Study the drawing (mm; zero at the part's minimum x, y, z) and answer. A direction names the side the tool comes from. Round coordinates to 2 decimals unless told otherwise and drop trailing zeros. Write each loop counter-clockwise with the first axis right and the second up, starting at its lowest first coordinate (ties: lowest second). Pieces come first, ordered by that corner, then holes.
(1) A cutting plane is placed at B-B, the plane x = 83. Give the vertices of the cut face in (y, z).
(2) For the marked faces 1, 2 and 3, determine the directions among +Z, -Z, +X, -X, +Y, -Y from which every point of the face is accessible in a straight line to the end or side of a thin tool.
(3) A cutting plane is placed at C-C, the plane z = 7.5. Give the vertices of the cut face in (x, y), and give its area (3 significant figures).
(4) A cutting plane is placed at D-D, the plane x = 113. Give the vertices of the cut face in (y, z), and give its area (3 significant figures).
(5) Find the intervals of material crossed by probe 1 along X at (y, z) = (61, 31.5); probe 2 along X at (y, z) = (65, 18); probe 3 along Z at (x, y) = (142, 99), in increasing order.
(6) The mould has two halves that part along Z. Classify the marked faces 4, 5, 6 and 7: +Z half, -Z half, draft (parallel to the pull), parting line (faces both ways), or undercut.
(7) Each of these flat-tipped pins is pushed along its axis until it touches: pin 1 Ø25 at (x, y) = (16, 94.5) entering from -Z; pin 2 Ø22 at (y, z) = (63, 36) entering from -X; pin 3 Ø6 at (y, z) = (88, 60.5) entering from +X. Where does it stop, or does it pass through?
(8) A cutting plane is placed at A-A, the plane y = 96.5. Give the vertices of the cut face in (x, z).
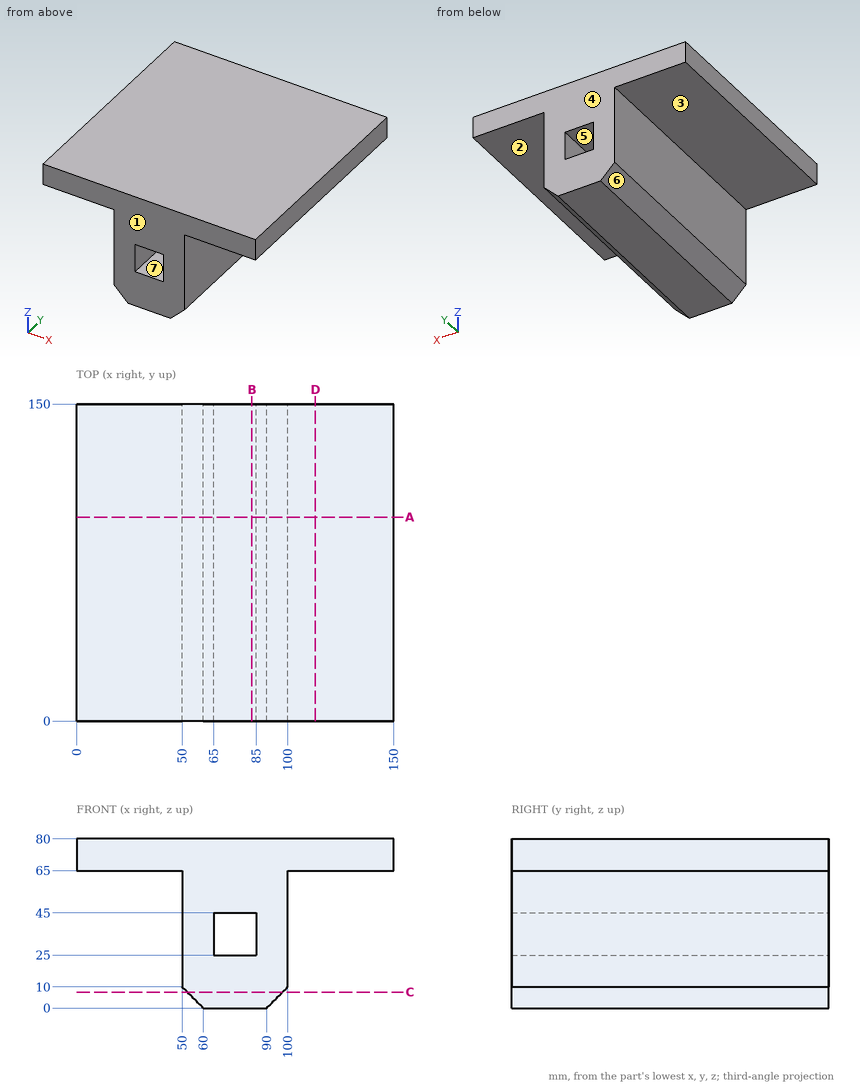
Solutions:
1. outline: (0, 0) - (150, 0) - (150, 25) - (0, 25) - close; (0, 45) - (150, 45) - (150, 80) - (0, 80) - close
2. face 1: +Z, -Z, +X, -X, -Y
2. face 2: -Z, +X, +Y, -Y
2. face 3: -Z, -X, +Y, -Y
3. outline: (52.5, 0) - (97.5, 0) - (97.5, 150) - (52.5, 150) - close
3. area: 6,750 mm2
4. outline: (0, 65) - (150, 65) - (150, 80) - (0, 80) - close
4. area: 2,250 mm2
5. probe 1: x = 50 to 65, 85 to 100
5. probe 2: x = 50 to 100
5. probe 3: z = 65 to 80
6. face 4: draft
6. face 5: undercut
6. face 6: -Z half
6. face 7: undercut
7. pin 1: stops at z = 65
7. pin 2: stops at x = 50
7. pin 3: stops at x = 100
8. outline: (0, 65) - (50, 65) - (50, 10) - (60, 0) - (90, 0) - (100, 10) - (100, 65) - (150, 65) - (150, 80) - (0, 80) - close; hole (65, 25) - (85, 25) - (85, 45) - (65, 45) - close
